```python
from build123d import *

# Parameters (mm, degrees)
BOSS_EXTRUDE1_DEPTH = 5
SKETCH3_W           = 2.8
SKETCH3_H           = 2.8
BOSS_EXTRUDE2_DEPTH = 5
SKETCH4_W           = 2.8
SKETCH4_H           = 2.8
BOSS_EXTRUDE3_DEPTH = 5


with BuildPart() as part:
    # Sketch2 → Boss-Extrude1 (new body)
    with BuildSketch(Plane.XY):
        with BuildLine():
            Line((4, 2.573223097), (-4.169337614, 2.573223097))
            ThreePointArc((-4.169337614, 2.573223097), (-5.169337614, 3.573223097), (-4.169337614, 4.573223097))
            Line((-4.169337614, 4.573223097), (-5, 4.573223097))
            ThreePointArc((-5, 4.573223097), (-5.39203954, 3.131635053), (-4.169337614, 2.273223097))
            Line((-4.169337614, 2.273223097), (4, 2.273223097))
            ThreePointArc((4, 2.273223097), (4.7, 1.573223097), (4, 0.873223097))
            Line((4, 0.873223097), (-4, 0.873223097))
            ThreePointArc((-4, 0.873223097), (-5.3, -0.426776903), (-4, -1.726776903))
            Line((-4, -1.726776903), (4, -1.726776903))
            ThreePointArc((4, -1.726776903), (4.7, -2.426776903), (4, -3.126776903))
            Line((4, -3.126776903), (-4, -3.126776903))
            ThreePointArc((-4, -3.126776903), (-5.3, -4.426776903), (-4, -5.726776903))
            Line((-4, -5.726776903), (4, -5.726776903))
            ThreePointArc((4, -5.726776903), (4.7, -6.426776903), (4, -7.126776903))
            Line((4, -7.126776903), (-5, -7.126776903))
            Line((-5, -7.126776903), (-5, -7.426776903))
            Line((-5, -7.426776903), (4, -7.426776903))
            ThreePointArc((4, -7.426776903), (5, -6.426776903), (4, -5.426776903))
            Line((4, -5.426776903), (-4, -5.426776903))
            ThreePointArc((-4, -5.426776903), (-5, -4.426776903), (-4, -3.426776903))
            Line((-4, -3.426776903), (4, -3.426776903))
            ThreePointArc((4, -3.426776903), (5, -2.426776903), (4, -1.426776903))
            Line((4, -1.426776903), (-4, -1.426776903))
            ThreePointArc((-4, -1.426776903), (-5, -0.426776903), (-4, 0.573223097))
            Line((-4, 0.573223097), (4, 0.573223097))
            ThreePointArc((4, 0.573223097), (5, 1.573223097), (4, 2.573223097))
        make_face()
        Polygon((-5, 4.573223097), (-4.169337614, 4.573223097), (5, 4.573223097), (5, 6.573223097), (-5, 6.573223097), align=None)
        Polygon((5, -7.426776903), (4, -7.426776903), (-5, -7.426776903), (-5, -9.426776903), (5, -9.426776903), align=None)
    extrude(amount=BOSS_EXTRUDE1_DEPTH)

    # Sketch3 → Boss-Extrude2 (add)
    with BuildSketch(Plane(origin=(0, 6.573223097, 0), x_dir=(1, 0, 0), z_dir=(0, 1, 0))):
        with Locations((0, -2.5)):
            Rectangle(SKETCH3_W, SKETCH3_H)
    extrude(amount=BOSS_EXTRUDE2_DEPTH)

    # Sketch4 → Boss-Extrude3 (add)
    with BuildSketch(Plane.XZ.offset(9.426776903)):
        with Locations((0, 2.5)):
            Rectangle(SKETCH4_W, SKETCH4_H)
    extrude(amount=BOSS_EXTRUDE3_DEPTH)


solid = part.part
```
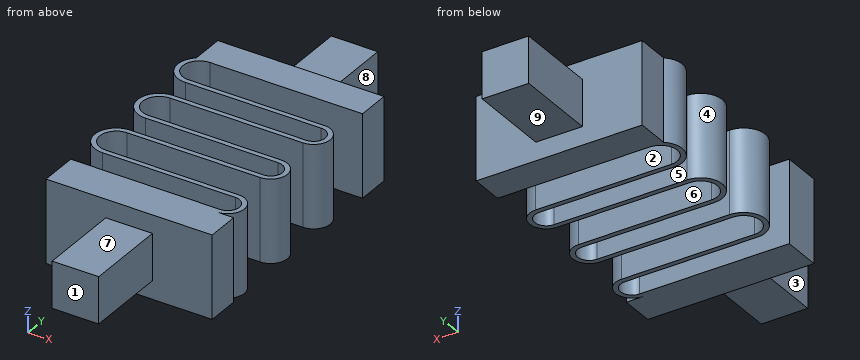
Verification items for the finished model (mm, model axes). Face numbers are marked on the shaded views. A direction names the side the tool comes from. Give positions to 0.01 mm unless a question says otherwise; leave off trailing zeros. Order: outer loops, then holes, each group sorted by start corner. A loop starts at its lowest first (then second) coordinate and runs counter-clockwise, first axis right, second up. Notation, with made-up numbers: M -9.5,-20.5 L 15.5,-20.5 A29 ccw 15.5,15.5 Z; hole C -34,44 d7. An arc over 180 degrees is marked long. Return JSON: item names as keys, results as strings. Group by question number.
1) Section check B-B on y = 1.75. Record the cut outline in (x, z), and give its area (3 significant figures).
2) Scan lines: line 1 (X direction, y = -2.5, z = 4.6); line 2 (X direction, y = 7, z = 1.4); line 3 (Z direction, x = -0.5, y = 9.25). Record each from-to range of solid material in increasing order.
3) Access from +Z, -Z, +X, -X, +Y, -Y to the whole of each face (thin tool, end or side, straight path). Record for the marked faces 5, 6, 7, 8 and 9.
4) Mould release check, pull along Y, two halves, no side actions. Record for the marked faces 1, 2, 3 and 4: pulls with the +Y half, pulls with the -Y half, needs draft (parallel to the pull), parting line crosses it, or undercut.
5) Go/stop test with flat-tipped pins: pin 1 Ø3 at (x, y) = (0, 8.5) entering from +Z; pin 2 Ø1.5 at (y, z) = (-4, 3) entering from -X; pin 3 Ø2 at (x, y) = (-0.5, 8) entering from -Z. Record where each tip stops, or that it passes through.
6) Section check A-A on y = 5.5. Record the cut outline in (x, z), and give its area (3 significant figures).
Answer block:
{
 "1": {"outline": "M 4.68,0 L 4.98,0 L 4.98,5 L 4.68,5 Z", "area": "1.53 mm^2"},
 "2": {"line 1": "x = 4.7 to 5", "line 2": "x = -1.4 to 1.4", "line 3": "z = 1.1 to 3.9"},
 "3": {"face 5": "+Z, -Z, -X", "face 6": "+Z, -Z, +X", "face 7": "+Z, +X, -X, -Y", "face 8": "+Z, -Z, +X, +Y", "face 9": "-Z, +X, -X, +Y"},
 "4": {"face 1": "pulls with the -Y half", "face 2": "undercut", "face 3": "needs draft", "face 4": "undercut"},
 "5": {"pin 1": "stops at z = 3.9", "pin 2": "stops at x = -5.3", "pin 3": "stops at z = 1.1"},
 "6": {"outline": "M -5,0 L 5,0 L 5,5 L -5,5 Z", "area": "50.0 mm^2"}
}
